Verification items for the finished model (mm, model axes). Give positions to 0.01 mm unless a question says otherwise; leave off trailing zeros. Loops run counter-clockwise (first coordinate to the right, second up) from the corner with the lowest first, then second, coordinate; pieces in that order, holes last. Notation, with made-up numbers: (40, 15.5) - (51, 15.5) arc R18 cw to (51, 32.5) - close; hole circle Ø8 at (-38, 86.5). An arc over 180 degrees is marked (long way). One line per question, with ' | ' between items. Start each with the question number.
1. Section check A-A, the plane z = 10. Enter the section's corners in (x, y), then the cut area to 3 significant figures.
2. Depth check by flat-ended pin: pin 1 Ø1 at (y, z) = (-251.5, 14.5) entering from -X; pin 2 Ø1.5 at (x, y) = (-23, -67) entering from -Z; pin 3 Ø3 at (x, y) = (-16.5, -139) entering from -Z. Enter the tip coordinate at first touch or a pass-through.
3. Thickness scan on line 1 along Y through (x, z) = (-45, 19); line 2 along Z through (x, y) = (19.5, -133.5); line 3 along X through (y, z) = (-415, -17). Record the ranges inside material, lowest first. Write a range as from..to.
4. Section check B-B, the plane y = 278.5. Enter the section's corners in (x, z), then the cut area to 3 significant figures.
5. Section check C-C, the plane x = -21. Enter the section's corners in (y, z), then the cut area to 3 significant figures.
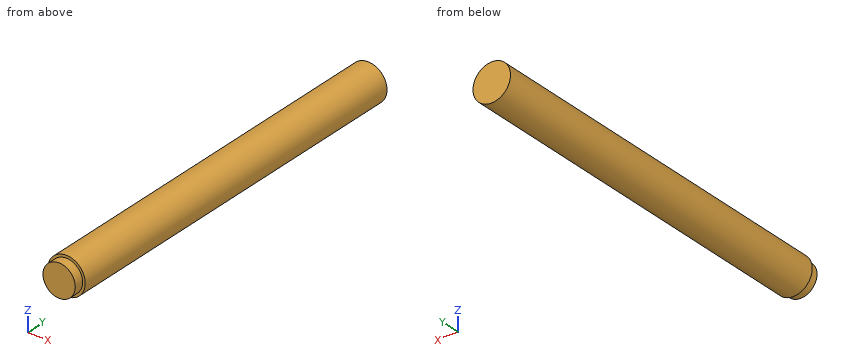
from build123d import *

# Parameters (mm, degrees)
F0_R      = 50
F1_DEPTH  = 500
F2_R      = 44.431358
F1_FACE_R = 50
F3_DEPTH  = 25
F4_R      = 43.104754
F5_DEPTH  = 25


with BuildPart() as f1:
    # F0 (on Front) → F1 (new body, symmetric)
    with BuildSketch(Plane.XZ):
        Circle(F0_R)
    extrude(amount=F1_DEPTH, both=True)

    # F2 (on Front) + F1_face (on face) → F3 (join)
    with BuildSketch(Plane.XZ):
        Circle(F2_R)
    with BuildSketch(Plane.XZ.offset(500)):
        Circle(F1_FACE_R)
    extrude(amount=F3_DEPTH)

    # F4 (on face) → F5 (join)
    with BuildSketch(Plane.XZ.offset(525)):
        Circle(F4_R)
    extrude(amount=F5_DEPTH)


solid = f1.part
Results list:
1) outline: (-48.99, -525) - (-41.93, -525) - (-41.93, -550) - (41.93, -550) - (41.93, -525) - (48.99, -525) - (48.99, 500) - (-48.99, 500) - close | area: 103,000 mm²
2) pin 1: x = -48 | pin 2: z = -44.78 | pin 3: z = -47.7
3) line 1: -525..500 | line 2: -46.04..46.04 | line 3: -47.02..47.02
4) outline: circle Ø100 at (0, 0) | area: 7,850 mm²
5) outline: (-550, -37.64) - (-525, -37.64) - (-525, -45.38) - (500, -45.38) - (500, 45.38) - (-525, 45.38) - (-525, 37.64) - (-550, 37.64) - close | area: 94,900 mm²
